Check sheet for the modelled part. Datum: model origin and axes. Units: mm. Give positions to 0.01 mm unless a question says otherwise; leave off trailing zeros. Loops run counter-clockwise (first coordinate to the right, second up) from the corner with the lowest first, then second, coordinate; pieces in that order, holes last. Notation, with made-up numbers: (55, 45) -> (71, 45) arc R14 ccw to (71, 62) -> close; hole circle Ø11 at (-9.75, 87.5). An arc over 180 degrees is marked (long way). Write each question's results on one line, items separated by ' | '. Start each with the question number.
Item 1: Mould release check, pull along Y, two halves, no side actions. Record for faces 1 (the face through (0, 498, -8)), 2 (the face through (0.31, 641.92, -521.93)), 3 (the face through (0.313, 427.142, 490.998)), 4 (the face through (0.31, 641.92, 494.07)): pulls with the +Y half, pulls with the -Y half, needs draft (parallel to the pull), parting line crosses it, or undercut.
Item 2: Cross-section at D-D on z = 211.5. Enter the section's corners in (x, y) (3 decimals).
Item 3: Cross-section at B-B on x = 0.35. Enter the section's corners in (y, z).
Item 4: Scan lines: line 1 along Z through (x, y) = (0.4, 647.7); line 2 along Z through (x, y) = (0.5, 642); line 3 along Y through (x, z) = (0.2, -508). Record each from-to range of solid material in increasing order.
Item 5: Cross-section at C-C on z = 508. Enter the section's corners in (x, y) (3 decimals).
Item 6: Gauge pin test, flat end, axial feed: pin 1 Ø24 at (y, z) = (647.7, 508) entering from -X (1 decimal). Record the tip position at first contact, or that the pin passes through.
Item 7: Cross-section at A-A on y = 647.7. Enter the section's corners in (x, z) (3 decimals), then the cut area to 3 significant figures.
from build123d import *

# Parameters (mm, degrees)
SKETCH1_R           = 15.08125
BOSS_EXTRUDE1_DEPTH = 0.635
FILLET1_R           = 12.7


with BuildPart() as part:
    # Sketch1 → Boss-Extrude1 (new body)
    with BuildSketch(Plane(origin=(0, 0, 0), x_dir=(0, 0, -1), z_dir=(1, 0, 0))):
        with BuildLine():
            Line((-558.8, 609.6), (-558.8, 685.8))
            Line((-558.8, 685.8), (558.8, 685.8))
            Line((558.8, 685.8), (558.8, 609.6))
            ThreePointArc((558.8, 609.6), (492.779998657, 429.230002015), (325.91999876, 334.100000517))
            Line((325.91999876, 334.100000517), (152.4, 304.8))
            Line((152.4, 304.8), (-152.4, 304.8))
            Line((-152.4, 304.8), (-325.91999876, 334.100000517))
            ThreePointArc((-325.91999876, 334.100000517), (-492.779998657, 429.230002015), (-558.8, 609.6))
        make_face()
        with Locations((-508, 647.7)):
            Circle(SKETCH1_R, mode=Mode.SUBTRACT)
        with Locations((508, 647.7)):
            Circle(SKETCH1_R, mode=Mode.SUBTRACT)
    extrude(amount=BOSS_EXTRUDE1_DEPTH)

    # Fillet1
    fillet1_edges = [part.edges().sort_by_distance(p)[0] for p in [
        (0.3175, 304.8, -152.4),
        (0.3175, 304.8, 152.4),
        (0.3175, 685.8, 558.8),
        (0.3175, 685.8, -558.8),
    ]]
    fillet(fillet1_edges, radius=FILLET1_R)


solid = part.part
Answer sheet:
1) face 1: needs draft | face 2: undercut | face 3: pulls with the -Y half | face 4: undercut
2) outline: (0, 314.779) -> (0.635, 314.779) -> (0.635, 685.8) -> (0, 685.8) -> close
3) outline: (304.8, -151.34) arc R12.7 ccw to (304.98, -153.45) -> (334.1, -325.92) arc R279.4 ccw to (609.6, -558.8) -> (673.1, -558.8) arc R12.7 ccw to (685.8, -546.1) -> (685.8, 546.1) arc R12.7 ccw to (673.1, 558.8) -> (609.6, 558.8) arc R279.4 ccw to (334.1, 325.92) -> (304.98, 153.45) arc R12.7 ccw to (304.8, 151.34) -> close; hole circle Ø30.16 at (647.7, -508); hole circle Ø30.16 at (647.7, 508)
4) line 1: z = -558.8 to -523.08, -492.92 to 492.92, 523.08 to 558.8 | line 2: z = -558.8 to -521.96, -494.04 to 494.04, 521.96 to 558.8 | line 3: y = 448.96 to 632.62, 662.78 to 685.8
5) outline: (0, 448.956) -> (0.635, 448.956) -> (0.635, 632.619) -> (0, 632.619) -> close; (0, 662.781) -> (0.635, 662.781) -> (0.635, 685.8) -> (0, 685.8) -> close
6) pin 1: passes through
7) outline: (0, -558.8) -> (0.635, -558.8) -> (0.635, -523.081) -> (0, -523.081) -> close; (0, -492.919) -> (0.635, -492.919) -> (0.635, 492.919) -> (0, 492.919) -> close; (0, 523.081) -> (0.635, 523.081) -> (0.635, 558.8) -> (0, 558.8) -> close | area: 671 mm²
